```python
from build123d import *

# Parameters (mm, degrees)
F4_DEPTH = 30.001
F5_W     = 6
F5_H     = 7
F6_DEPTH = 13


with BuildPart() as f1:
    # F0 (on Right) → F1 (revolve)
    with BuildSketch(Plane.YZ):
        with BuildLine():
            Line((-30, 0), (0, 0))
            ThreePointArc((0, 0), (-15, 15), (-30, 0))
        make_face()
    revolve(axis=Axis((0, -15, 0), (0, -1, 0)))

    # F3 (on offset) → F4 (cut, through all)
    with BuildSketch(Plane.XY.offset(15)):
        with BuildLine():
            Line((15, 0), (0, 0))
            Line((0, 0), (-15, 0))
            ThreePointArc((-15, 0), (0, -3), (15, 0))
        make_face()
    extrude(amount=-F4_DEPTH, mode=Mode.SUBTRACT)

    # F5 (on Front) → F6 (cut)
    with BuildSketch(Plane.XZ):
        Rectangle(F5_W, F5_H)
    extrude(amount=F6_DEPTH, mode=Mode.SUBTRACT)


solid = f1.part
```
CAD build for the part. Positions are in the model's coordinates, mm. A direction names the side the tool comes from. Round coordinates to 2 decimals unless told otherwise and drop trailing zeros. Loops run counter-clockwise (first coordinate to the right, second up) from the corner with the lowest first, then second, coordinate; pieces in that order, holes last. Notation, with made-up numbers: M 79.25,54.5 L 110.25,54.5 A11 ccw 110.25,74.5 Z; hole C -13.5,52 d3. An arc over 180 degrees is marked long. Use a Markdown table: item, result. Add a question column.
(1) Flat gauge pins, fed straight in: pin 1 (1 mm diameter, centred on y = -21.5, z = -12, fed in from +X); pin 2 (8 mm diameter, centred on y = -20.5, z = 2, fed in from +X); pin 3 (3 mm diameter, centred on x = -0.5, z = 1, fed in from +Y). Where does each tip first touch, or does it go through?
(2) Cut at C-C (z = -1.25). Give the cut face in (x, y), and give its area (3 significant figures).
(3) Cut at D-D (y = -16). Give the cut face in (x, z), and give its area (3 significant figures).
(4) Which spindle directions (+Z, -Z, +X, -X, +Y, -Y) get a long thin tool onto all of the face, cutting with end or side? Do faces 1 (the face through (0, -8, -3.5)), 2 (the face through (3.386, -2.853, 0.126)). Say none if no direction does.
(5) Cut at B-B (x = 2.5). Give the cut face in (y, z).
(6) Drill centre lines: line 1 (Z direction, x = 5.5, y = -15); line 2 (Y direction, x = -1, z = 12); line 3 (X direction, y = -16.25, z = -0.75). Where is each one in solid material? Low to high.
(7) Cut at A-A (y = -12). Give the cut face in (x, z).
Geometry says:
| question | item | result |
|---|---|---|
| 1 | pin 1 | stops at x = 7.22 |
| 1 | pin 2 | stops at x = 14.89 |
| 1 | pin 3 | stops at y = -13 |
| 2 | outline | M -7.75,-2.22 A14.95 ccw long 7.75,-2.22 A39 cw 3,-2.88 L 3,-13 L -3,-13 L -3,-2.88 A39 cw Z |
| 2 | area | 611 mm² |
| 3 | outline | C 0,0 d29.93 |
| 3 | area | 704 mm² |
| 4 | face 1 | +Y |
| 4 | face 2 | +Z, -Z, +Y |
| 5 | outline | M -13,-3.5 L -13,3.5 L -2.92,3.5 L -2.92,8.53 A14.79 ccw long -2.92,-8.53 L -2.92,-3.5 Z |
| 6 | line 1 | z = -13.96 to 13.96 |
| 6 | line 2 | y = -23.94 to -6.06 |
| 6 | line 3 | x = -14.93 to 14.93 |
| 7 | outline | C 0,0 d29.39; hole M -3,-3.5 L 3,-3.5 L 3,3.5 L -3,3.5 Z |
